For this review, take the finished solid that the model builds, in its own axes (mm). A direction names the side the tool comes from. Round coordinates to 2 decimals unless told otherwise and drop trailing zeros. Write each loop counter-clockwise with the first axis right and the second up, starting at its lowest first coordinate (ties: lowest second). Pieces come first, ordered by that corner, then holes. Notation, with made-up numbers: (-25.5, 47) -> (28.5, 47) arc R16 ccw to (28.5, 68) -> close; hole circle Ø9 at (62, -21.5). An arc over 180 degrees is marked (long way). Write each question's results on one line, items separated by ' | '. Start each with the question number.
Item 1: Add section D-D (y = 1). State the section outline as (x, z) points, plus the area to 3 significant figures.
Item 2: Add section C-C (x = -6). State the section outline as (y, z) points.
Item 3: The part is to be moulded in two halves that separate along Y. For faces 1 (the flat face through (-3, -11, -20)), 2 (the cylindrical face through (-4.101, 31.232, 27.521)), 3 (the cylindrical face through (0.32, 11.91, 8.47)), say which applies: +Y half, -Y half, draft (parallel to the pull), parting line (faces both ways), or undercut.
Item 4: To check wall thickness, follow line 1 along Y through (x, z) = (0, -7); line 2 along Y through (x, z) = (0, 7.75); line 3 along Z through (x, y) = (-5.5, -5.5). State the ranges of each line that lie inside material, in increasing order.
Item 5: Add section A-A (z = 0). State the section outline as (x, y) points.
Item 6: Clearance check with flat-ended pins moving along their axes: pin 1 (5.5 mm diameter, centred on x = 4, z = 20, fed in from -Y); pin 2 (0.6 mm diameter, centred on y = 17, z = 22, fed in from +X); pin 3 (2 mm diameter, centred on x = -11, z = 3.5, fed in from +Y); pin 4 (7.5 mm diameter, centred on x = -7, z = 18.5, fed in from -Y). State where each tip first meets the part, or that it passes through.
Item 7: Tool access review of faces 4 (the flat face through (-2, -17, 20)), 5 (the flat face through (14, -14, 29)), 6 (the flat face through (7, 26, 26)): name each direction out of +Z, -Z, +X, -X, +Y, -Y from which nothing blocks a thin tool from reaching the whole face with its end or side.
Item 8: Add section B-B (y = 9.5). State the section outline as (x, z) points.
from build123d import *

# Parameters (mm, degrees)
F3_DEPTH = 18
F4_D     = 4.86
F6_DEPTH = 26


with BuildPart() as f1:
    # F0 (on Front) → F1 (revolve)
    with BuildSketch(Plane.XZ):
        Polygon((0, 29), (0, 6), (26.5, 6), (26.5, 26), (31.5, 26), (31.5, 29), align=None)
    revolve(axis=Axis((0, 0, 14.5), (0, 0, 1)))

    # F2 (on face) → F3 (cut)
    with BuildSketch(Plane.XY.offset(29)):
        with BuildLine():
            Line((2, -16.1), (0, -16.1))
            Line((0, -16.1), (-2, -16.1))
            Line((-2, -16.1), (-2, -18.1903820741))
            ThreePointArc((-2, -18.1903820741), (0, -18.3), (2, -18.1903820741))
            Line((2, -18.1903820741), (2, -16.1))
        make_face()
        with BuildLine():
            Line((0, -9.5), (0, 0))
            Line((0, 0), (0, 9.5))
            Line((0, 9.5), (0, 16.1))
            Line((0, 16.1), (-2, 16.1))
            Line((-2, 16.1), (-8.6994252684, 16.1))
            ThreePointArc((-8.6994252684, 16.1), (-18.3, 0), (-8.6994252684, -16.1))
            Line((-8.6994252684, -16.1), (-2, -16.1))
            Line((-2, -16.1), (0, -16.1))
            Line((0, -16.1), (0, -9.5))
        make_face()
        with BuildLine():
            Line((-2, 16.1), (0, 16.1))
            Line((0, 16.1), (2, 16.1))
            Line((2, 16.1), (2, 18.1903820741))
            ThreePointArc((2, 18.1903820741), (0, 18.3), (-2, 18.1903820741))
            Line((-2, 18.1903820741), (-2, 16.1))
        make_face()
        with BuildLine():
            Line((0, 9.5), (0, 0))
            Line((0, 0), (10, 0))
            Line((10, 0), (18.3, 0))
            ThreePointArc((18.3, 0), (15.7176569884, 9.3725801567), (8.6994252684, 16.1))
            Line((8.6994252684, 16.1), (2, 16.1))
            Line((2, 16.1), (0, 16.1))
            Line((0, 16.1), (0, 9.5))
        make_face()
        with BuildLine():
            Line((10, 0), (0, 0))
            Line((0, 0), (0, -9.5))
            Line((0, -9.5), (0, -16.1))
            Line((0, -16.1), (2, -16.1))
            Line((2, -16.1), (8.6994252684, -16.1))
            ThreePointArc((8.6994252684, -16.1), (15.7176569884, -9.3725801567), (18.3, 0))
            Line((18.3, 0), (10, 0))
        make_face()
    extrude(amount=-F3_DEPTH, mode=Mode.SUBTRACT)

    # F4 (through all)
    with Locations(Plane.XY.offset(29)):
        with Locations((0, 9.5), (0, -9.5)):
            Hole(F4_D / 2)

    # F5 (on face) → F6 (join)
    with BuildSketch(Plane(origin=(0, 0, 6), x_dir=(1, 0, 0), z_dir=(0, 0, -1))):
        with BuildLine():
            ThreePointArc((4, 9.5), (0, 13.5), (-4, 9.5))
            ThreePointArc((-4, 9.5), (0, 5.5), (4, 9.5))
        make_face()
        with BuildLine():
            ThreePointArc((3, 9.5), (0, 6.5), (-3, 9.5))
            ThreePointArc((-3, 9.5), (0, 12.5), (3, 9.5))
        make_face(mode=Mode.SUBTRACT)
        with BuildLine():
            ThreePointArc((4, -9.5), (0, -5.5), (-4, -9.5))
            ThreePointArc((-4, -9.5), (0, -13.5), (4, -9.5))
        make_face()
        with BuildLine():
            ThreePointArc((3, -9.5), (0, -12.5), (-3, -9.5))
            ThreePointArc((-3, -9.5), (0, -6.5), (3, -9.5))
        make_face(mode=Mode.SUBTRACT)
    extrude(amount=F6_DEPTH)


solid = f1.part
Responses:
1) outline: (-31.48, 26) -> (-26.48, 26) -> (-26.48, 6) -> (26.48, 6) -> (26.48, 26) -> (31.48, 26) -> (31.48, 29) -> (18.27, 29) -> (18.27, 11) -> (-18.27, 11) -> (-18.27, 29) -> (-31.48, 29) -> close | area: 590 mm^2
2) outline: (-30.92, 26) -> (-25.81, 26) -> (-25.81, 6) -> (25.81, 6) -> (25.81, 26) -> (30.92, 26) -> (30.92, 29) -> (16.1, 29) -> (16.1, 11) -> (-16.1, 11) -> (-16.1, 29) -> (-30.92, 29) -> close
3) face 1: draft | face 2: parting line | face 3: undercut
4) line 1: y = -13.5 to -12.5, -6.5 to -5.5, 5.5 to 6.5, 12.5 to 13.5 | line 2: y = -26.5 to -11.93, -7.07 to 7.07, 11.93 to 26.5 | line 3: z = 6 to 11
5) outline: circle Ø8 at (0, -9.5); circle Ø8 at (0, 9.5); hole circle Ø6 at (0, -9.5); hole circle Ø6 at (0, 9.5)
6) pin 1: stops at y = -26.47 | pin 2: stops at x = 20.58 | pin 3: passes through | pin 4: stops at y = -26.3
7) face 4: +Z | face 5: +Z, +X, -X, +Y, -Y | face 6: -Z
8) outline: (-30.03, 26) -> (-24.74, 26) -> (-24.74, 6) -> (-4, 6) -> (-4, -20) -> (-3, -20) -> (-3, 6) -> (-2.43, 6) -> (-2.43, 11) -> (-15.64, 11) -> (-15.64, 29) -> (-30.03, 29) -> close; (2.43, 6) -> (3, 6) -> (3, -20) -> (4, -20) -> (4, 6) -> (24.74, 6) -> (24.74, 26) -> (30.03, 26) -> (30.03, 29) -> (15.64, 29) -> (15.64, 11) -> (2.43, 11) -> close
